Autodesk Inventor part; units mm, degrees
ref_plane "YZ Plane" through (0, 0, 0) normal (1, 0, 0) x (0, 1, 0)
ref_plane "XZ Plane" through (0, 0, 0) normal (0, 1, 0) x (-1, 0, 0)
ref_plane "XY Plane" through (0, 0, 0) normal (0, 0, 1) x (1, 0, 0)
sketch "Sketch1" plane through (0, 0, 0) normal (0, 0, 1) x (1, 0, 0)
  line L0 (-222.5, 72) -> (222.5, 72)
  line L1 (222.5, 72) -> (222.5, -72)
  line L2 (222.5, -72) -> (-222.5, -72)
  line L3 (-222.5, -72) -> (-222.5, 72)
  point P0 (0, 0)
  dimension "d0" = 445
  dimension "d1" = 144
  dimension "d2" = 72
  dimension "d3" = 222.5
extrude "Extrusion1" add sketch "Sketch1" along normal blind 8
hole "Hole1" at (-142.5, 0, 8) direction (0, 0, -1) diameter 22 end through all
sketch "Sketch2" plane through (0, 0, 8) normal (0, 0, 1) x (1, 0, 0)
  circle A0 centre (-142.5, 0) radius 11
  circle A1 centre (-142.5, 0) radius 14.5
  point P0 (0, 0)
  dimension "d15" = 29
extrude "Extrusion2" cut sketch "Sketch2" against normal blind 4
sketch "Sketch3" plane through (0, 0, 8) normal (0, 0, 1) x (1, 0, 0)
  line L0 (114.5, 23.5) -> (142.5, 23.5)
  line L1 (142.5, 23.5) -> (142.5, -23.5)
  line L2 (142.5, -23.5) -> (114.5, -23.5)
  line L3 (114.5, -23.5) -> (114.5, 23.5)
  line L4 (222.5, -72) -> (222.5, 72)
  point P0 (0, 0)
  dimension "d18" = 28
  dimension "d19" = 47
  dimension "d20" = 80
  dimension "d21" = 23.5
extrude "Extrusion3" cut sketch "Sketch3" against normal through all
properties part number "placa verticala priza"
Could you check a few things on this model? Use its own coordinates, in mm. A direction names the side the tool comes from. Round coordinates to 2 decimals unless told otherwise and drop trailing zeros. Write each loop counter-clockwise with the first axis right and the second up, starting at its lowest first coordinate (ties: lowest second). Pieces come first, ordered by that corner, then holes. Notation, with made-up numbers: (62, -39) - (116, -39) arc R25 cw to (116, -3) - close; hole circle Ø3 at (58.5, 37.5). An arc over 180 degrees is marked (long way). Use a Markdown table: item, result.
Q1. For pin 1 (23 mm diameter, centred on x = -142.5, y = 0, fed in from +Z), with a flat end and sliding along its axis, tell me the tip position at first contact or that it passes through.
Output values:
| item | result |
|---|---|
| pin 1 | z = 4 |
Q2. I want a section at C-C (x = -142.5). List the corners of the cut face in (y, z) for me.
Output values:
| item | result |
|---|---|
| outline | (-72, 0) - (-11, 0) - (-11, 4) - (-14.5, 4) - (-14.5, 8) - (-72, 8) - close; (11, 0) - (72, 0) - (72, 8) - (14.5, 8) - (14.5, 4) - (11, 4) - close |
Q3. For faces 4 (the cylindrical face through (-156.986, 0.638, 6.028)), 5 (the flat face through (-222.5, -1, 4)), 6 (the flat face through (128, 23.5, 4)), which set-ups out of +Z, -Z, +X, -X, +Y, -Y let a thin tool reach every point of the face, with its end or its side?
Output values:
| item | result |
|---|---|
| face 4 | +Z |
| face 5 | +Z, -Z, -X, +Y, -Y |
| face 6 | +Z, -Z |
Q4. I want a section at A-A (y = 0). List the corners of the cut face in (x, z) for me.
Output values:
| item | result |
|---|---|
| outline | (-222.5, 0) - (-153.5, 0) - (-153.5, 4) - (-157, 4) - (-157, 8) - (-222.5, 8) - close; (-131.5, 0) - (114.5, 0) - (114.5, 8) - (-128, 8) - (-128, 4) - (-131.5, 4) - close; (142.5, 0) - (222.5, 0) - (222.5, 8) - (142.5, 8) - close |
Q5. I want a section at D-D (y = 19.5). List the corners of the cut face in (x, z) for me.
Output values:
| item | result |
|---|---|
| outline | (-222.5, 0) - (114.5, 0) - (114.5, 8) - (-222.5, 8) - close; (142.5, 0) - (222.5, 0) - (222.5, 8) - (142.5, 8) - close |
Q6. Thinking about a two-plate mould opening in Y: for faces 1 (the flat face through (222.5, 1, 4)), 2 (the flat face through (-145, 11, 4)), 3 (the flat face through (3, -72, 4)), which applies, released by +Y, released by -Y, zero draft, split by the parting line, or undercut?
Output values:
| item | result |
|---|---|
| face 1 | zero draft |
| face 2 | undercut |
| face 3 | released by -Y |
Q7. Please list where these lines run through material, in increasing order: L1, parallel to X at y = 0, z = 2.25; L2, parallel to X at y = 2, z = 7; L3, parallel to Y at x = -142.5, z = 5.2.
Output values:
| item | result |
|---|---|
| L1 | -222.5 to -153.5, -131.5 to 114.5, 142.5 to 222.5 |
| L2 | -222.5 to -156.86, -128.14 to 114.5, 142.5 to 222.5 |
| L3 | -72 to -14.5, 14.5 to 72 |
Q8. I want a section at B-B (z = 5.25). List the corners of the cut face in (x, y) for me.
Output values:
| item | result |
|---|---|
| outline | (-222.5, -72) - (222.5, -72) - (222.5, 72) - (-222.5, 72) - close; hole circle Ø29 at (-142.5, 0); hole (114.5, -23.5) - (142.5, -23.5) - (142.5, 23.5) - (114.5, 23.5) - close |
